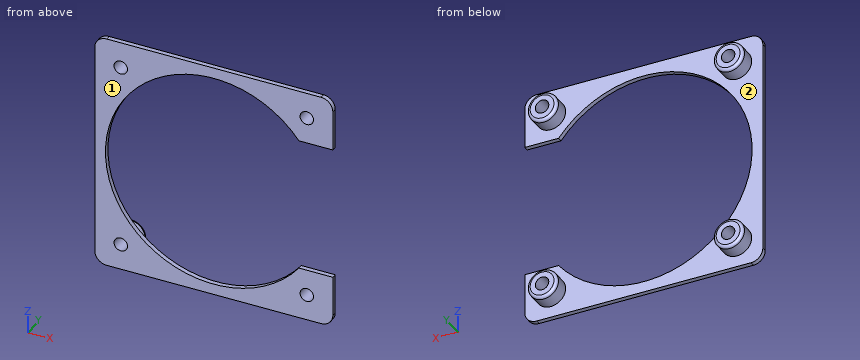
from build123d import *

# Parameters (mm, degrees)
F1_DEPTH = 1.016
F2_R     = 3.175
F3_DEPTH = 3.6322
F5_D     = 2.8702
F6_R     = 0.635


with BuildPart() as f1:
    # F0 (on Front) → F1 (new body)
    with BuildSketch(Plane.XZ):
        with BuildLine():
            ThreePointArc((0, 2.54), (0.7439487758, 0.7439487758), (2.54, 0))
            Line((2.54, 0), (48.26, 0))
            ThreePointArc((48.26, 0), (50.0560512242, 0.7439487758), (50.8, 2.54))
            Line((50.8, 2.54), (50.8, 11.1125))
            Line((50.8, 11.1125), (43.5693241413, 11.1125))
            ThreePointArc((43.5693241413, 11.1125), (2.286, 25.4), (43.5693241413, 39.6875))
            Line((43.5693241413, 39.6875), (50.8, 39.6875))
            Line((50.8, 39.6875), (50.8, 48.26))
            ThreePointArc((50.8, 48.26), (50.0560512242, 50.0560512242), (48.26, 50.8))
            Line((48.26, 50.8), (2.54, 50.8))
            ThreePointArc((2.54, 50.8), (0.7439487758, 50.0560512242), (0, 48.26))
            Line((0, 48.26), (0, 2.54))
        make_face()
    extrude(amount=F1_DEPTH)

    # F2 (on face) → F3 (join)
    with BuildSketch(Plane(origin=(0, 0, 0), x_dir=(-1, 0, 0), z_dir=(0, 1, 0))):
        with Locations((-45.2501, 45.2501)):
            Circle(F2_R)
        with Locations((-5.5499, 45.2501)):
            Circle(F2_R)
        with Locations((-5.5499, 5.5499)):
            Circle(F2_R)
        with Locations((-45.2501, 5.5499)):
            Circle(F2_R)
    extrude(amount=F3_DEPTH)

    # F5 (through all)
    with Locations(Plane(origin=(0, 3.6322, 0), x_dir=(-1, 0, 0), z_dir=(0, 1, 0))):
        with Locations((-45.2501, 45.2501), (-5.5499, 45.2501), (-5.5499, 5.5499), (-45.2501, 5.5499)):
            Hole(F5_D / 2)

    # F6
    f6_edges = [f1.edges().sort_by_distance(p)[0] for p in [
        (48.4251, 3.6322, 45.2501),
        (8.7249, 3.6322, 45.2501),
        (8.7249, 3.6322, 5.5499),
        (48.4251, 3.6322, 5.5499),
    ]]
    fillet(f6_edges, radius=F6_R)


solid = f1.part
The model under review builds one solid part; all positions refer to its coordinate system, in mm. Face numbers are marked on the shaded views. Round coordinates to 2 decimals unless told otherwise and drop trailing zeros. Order: outer loops, then holes, each group sorted by start corner. A loop starts at its lowest first (then second) coordinate and runs counter-clockwise, first axis right, second up. Notation, with made-up numbers: (46, 20) -> (71, 20) arc R21 cw to (71, 55) -> close; hole circle Ø11 at (68, 0.25). An arc over 180 degrees is marked (long way). Return JSON: item names as keys, results as strings.
1. Take a section at C-C (x = 12.5). Write out the cut boundary in (y, z), then the cut area to 3 significant figures.
Answer block:
{"outline": "(-1.02, 0) -> (0, 0) -> (0, 6.22) -> (-1.02, 6.22) -> close; (-1.02, 44.58) -> (0, 44.58) -> (0, 50.8) -> (-1.02, 50.8) -> close", "area": "12.6 mm²"}
2. Take a section at A-A (x = 25.4). Write out the cut boundary in (y, z).
Answer block:
{"outline": "(-1.02, 0) -> (0, 0) -> (0, 2.29) -> (-1.02, 2.29) -> close; (-1.02, 48.51) -> (0, 48.51) -> (0, 50.8) -> (-1.02, 50.8) -> close"}
3. Take a section at D-D (z = 25.4). Write out the cut boundary in (x, y).
Answer block:
{"outline": "(0, -1.02) -> (2.29, -1.02) -> (2.29, 0) -> (0, 0) -> close"}
4. The part is to be moulded in two halves that separate along X. For the marked faces 1 and 2, say which applies: +X half, -X half, draft (parallel to the pull), parting line (faces both ways), or undercut.
Answer block:
{"face 1": "draft", "face 2": "undercut"}
5. Take a section at B-B (y = 2.05). Write out the cut boundary in (x, z) (3 decimals).
Answer block:
{"outline": "circle Ø6.35 at (5.55, 5.55); circle Ø6.35 at (5.55, 45.25); circle Ø6.35 at (45.25, 5.55); circle Ø6.35 at (45.25, 45.25); hole circle Ø2.87 at (5.55, 5.55); hole circle Ø2.87 at (5.55, 45.25); hole circle Ø2.87 at (45.25, 5.55); hole circle Ø2.87 at (45.25, 45.25)"}
6. For L1, parallel to Z at x = 46, y = 3.25; L2, parallel to Z at x = 25.4, y = -0.65; L3, parallel to Y at x = 36.5, z = 46, list the stretches that pass through material, from the lowest coordinate up. Write a range as [from, to].
Answer block:
{"L1": "z = [2.52, 4.33], [6.77, 8.58], [42.22, 44.03], [46.47, 48.28]", "L2": "z = [0, 2.29], [48.51, 50.8]", "L3": "y = [-1.02, 0]"}
